Read the model definition and answer for the solid it produces. Units are mm, in the model's axes. Face numbers are marked on the shaded views. A direction names the side the tool comes from. Give positions to 0.01 mm unless a question says otherwise; leave off trailing zeros. Order: outer loops, then holes, each group sorted by start corner. A loop starts at its lowest first (then second) coordinate and runs counter-clockwise, first axis right, second up. Notation, with made-up numbers: (43.25, -39.5) - (69.25, -39.5) arc R27 ccw to (69.25, -22.5) - close; hole circle Ø8 at (-18, 22.25). An arc over 180 degrees is marked (long way). One line per item, written item: value. Start each with the question number.
```python
from build123d import *

# Parameters (mm, degrees)
SKETCH2_W               = 6.03
SKETCH2_H               = 7
BOSS_EXTRUDE1_DEPTH     = 15.64
CUT_EXTRUDE1_DEPTH      = 17.307968144
CUT_EXTRUDE1_DEPTH_BACK = 17.307968144
SKETCH3_W               = 4
SKETCH3_H               = 8.3
FILLET1_R               = 3.5
SKETCH4_R               = 1.5
BOSS_EXTRUDE2_DEPTH     = 4
CUT_EXTRUDE2_DEPTH      = 18.398270747
CUT_EXTRUDE2_DEPTH_BACK = 18.398270747
SKETCH7_W               = 7
SKETCH7_H               = 1.3
BOSS_EXTRUDE3_DEPTH     = 0.4
SKETCH8_R               = 1.75
BOSS_EXTRUDE4_DEPTH     = 21.14
SKETCH9_R               = 3.35
BOSS_EXTRUDE5_DEPTH     = 1.1
BOSS_EXTRUDE6_DEPTH     = 10.1
SKETCH11_R              = 3.35
BOSS_EXTRUDE7_DEPTH     = 1.1
SKETCH12_R              = 1.175
BOSS_EXTRUDE8_DEPTH     = 1
SKETCH13_R              = 1.25
BOSS_EXTRUDE9_DEPTH     = 1
CHAMFER1_SIZE           = 0.5
CHAMFER1_SIZE2          = 0.595876796
SKETCH14_R              = 2.55
BOSS_EXTRUDE10_DEPTH    = 0.5
CHAMFER3_SIZE           = 0.3


with BuildPart() as part:
    # Sketch2 → Boss-Extrude1 (new body)
    with BuildSketch(Plane(origin=(0, 0, 0), x_dir=(1, 0, 0), z_dir=(0, 1, 0))):
        Rectangle(SKETCH2_W, SKETCH2_H)
    extrude(amount=BOSS_EXTRUDE1_DEPTH)

    # Sketch3 → Cut-Extrude1 (cut, two sides: drawn at the far end of the back side and taken through both)
    with BuildSketch(Plane.XY.offset(-CUT_EXTRUDE1_DEPTH_BACK)):
        with Locations((0, 4.15)):
            Rectangle(SKETCH3_W, SKETCH3_H)
    extrude(amount=CUT_EXTRUDE1_DEPTH + CUT_EXTRUDE1_DEPTH_BACK, mode=Mode.SUBTRACT)

    # Fillet1
    fillet1_edges = [part.edges().sort_by_distance(p)[0] for p in [
        (-2.5075, 0, 3.5),
        (-2.5075, 0, -3.5),
        (2.5075, 0, -3.5),
        (2.5075, 0, 3.5),
    ]]
    fillet(fillet1_edges, radius=FILLET1_R - 0.0001)  # a hair under: the kernel refuses the full size

    # Sketch4 → Boss-Extrude2 (add)
    with BuildSketch(Plane(origin=(-2, 0, 0), x_dir=(0, 0, -1), z_dir=(1, 0, 0))):
        with Locations(Location((0, 2.4, 0), (0, 0, 180))):
            Circle(SKETCH4_R)
    extrude(amount=BOSS_EXTRUDE2_DEPTH)

    # Sketch6 → Cut-Extrude2 (cut, two sides: drawn at the far end of the back side and taken through both)
    with BuildSketch(Plane(origin=(0, 0, -3.5), x_dir=(-1, 0, 0), z_dir=(0, 0, -1)).offset(-CUT_EXTRUDE2_DEPTH_BACK)):
        with BuildLine():
            Line((-0.25, 13.4336972), (-0.25, 13.9336972))
            Line((-0.25, 13.9336972), (0.25, 13.9336972))
            Line((0.25, 13.9336972), (0.25, 13.4336972))
            ThreePointArc((0.25, 13.4336972), (0, 9.6), (-0.25, 13.4336972))
        make_face()
    extrude(amount=CUT_EXTRUDE2_DEPTH + CUT_EXTRUDE2_DEPTH_BACK, mode=Mode.SUBTRACT)

    # Sketch7 → Boss-Extrude3 (add)
    with BuildSketch(Plane(origin=(3.015, 0, 0), x_dir=(0, 0, -1), z_dir=(1, 0, 0))):
        with Locations((0, 14.6)):
            Rectangle(SKETCH7_W, SKETCH7_H)
        with Locations((0, 10.35)):
            Rectangle(SKETCH7_W, SKETCH7_H)
    boss_extrude3 = extrude(amount=BOSS_EXTRUDE3_DEPTH)

    # Mirror1: Boss-Extrude3 across plane
    add(boss_extrude3.mirror(Plane(origin=(0, 0, 0), x_dir=(0, 0, 1), z_dir=(1, 0, 0))))

    # Sketch8 → Boss-Extrude4 (add)
    with BuildSketch(Plane(origin=(0, 15.64, 0), x_dir=(1, 0, 0), z_dir=(0, 1, 0))):
        with Locations(Location((0, 0, 0), (0, 0, 270))):
            Circle(SKETCH8_R)
    extrude(amount=BOSS_EXTRUDE4_DEPTH)

    # Sketch9 → Boss-Extrude5 (add)
    with BuildSketch(Plane(origin=(0, 36.78, 0), x_dir=(1, 0, 0), z_dir=(0, 1, 0))):
        with Locations(Location((0, 0, 0), (0, 0, 270))):
            Circle(SKETCH9_R)
    extrude(amount=BOSS_EXTRUDE5_DEPTH)

    # Sketch10 → Boss-Extrude6 (add)
    with BuildSketch(Plane(origin=(0, 37.88, 0), x_dir=(1, 0, 0), z_dir=(0, 1, 0))):
        Polygon((-0.55, 2.3), (-0.55, 0.55), (-2.3, 0.55), (-2.3, -0.55), (-0.55, -0.55), (-0.55, -2.3), (0.55, -2.3), (0.55, -0.55), (2.3, -0.55), (2.3, 0.55), (0.55, 0.55), (0.55, 2.3), align=None)
    extrude(amount=BOSS_EXTRUDE6_DEPTH)

    # Sketch11 → Boss-Extrude7 (add)
    with BuildSketch(Plane(origin=(0, 47.98, 0), x_dir=(1, 0, 0), z_dir=(0, 1, 0))):
        with Locations(Location((0, 0, 0), (0, 0, 270))):
            Circle(SKETCH11_R)
    extrude(amount=BOSS_EXTRUDE7_DEPTH)

    # Sketch12 → Boss-Extrude8 (add)
    with BuildSketch(Plane(origin=(0, 49.08, 0), x_dir=(1, 0, 0), z_dir=(0, 1, 0))):
        with Locations(Location((0, 0, 0), (0, 0, 270))):
            Circle(SKETCH12_R)
    extrude(amount=BOSS_EXTRUDE8_DEPTH)

    # Sketch13 → Boss-Extrude9 (add)
    with BuildSketch(Plane(origin=(0, 50.08, 0), x_dir=(1, 0, 0), z_dir=(0, 1, 0))):
        with Locations(Location((0, 0, 0), (0, 0, 270))):
            Circle(SKETCH13_R)
    extrude(amount=BOSS_EXTRUDE9_DEPTH)

    # Chamfer1
    chamfer1_edges = [part.edges().sort_by_distance(p)[0] for p in [
        (0, 51.08, -1.25),
    ]]
    chamfer1_side = [part.faces().sort_by_distance(p)[0] for p in [
        (0, 50.58, -1.25),
    ]]
    chamfer(chamfer1_edges, length=CHAMFER1_SIZE, length2=CHAMFER1_SIZE2, reference=chamfer1_side[0])

    # Sketch14 → Boss-Extrude10 (add)
    with BuildSketch(Plane(origin=(0, 15.64, 0), x_dir=(1, 0, 0), z_dir=(0, 1, 0))):
        with Locations(Location((0, 0, 0), (0, 0, 90))):
            Circle(SKETCH14_R)
    extrude(amount=BOSS_EXTRUDE10_DEPTH)

    # Chamfer3
    chamfer3_edges = [part.edges().sort_by_distance(p)[0] for p in [
        (0, 16.14, -1.75),
        (0, 16.14, 2.55),
    ]]
    chamfer(chamfer3_edges, length=CHAMFER3_SIZE)


solid = part.part
```
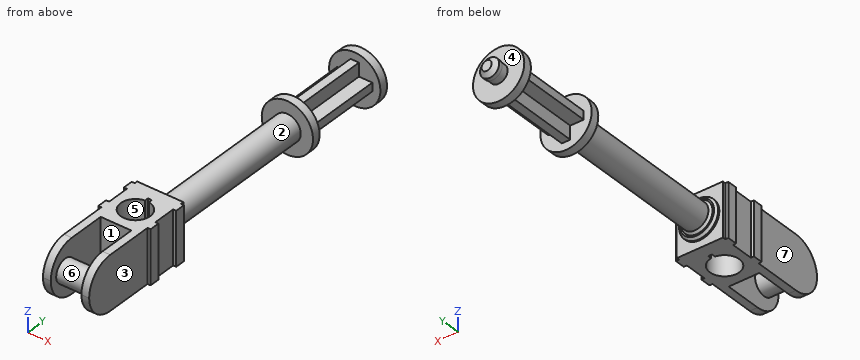
1) Section B-B on y = 40.5 is taken. Write down the section's boundary in (x, z).
2) Each of these flat-tipped pins is pushed along its axis until it touches: pin 1 (4 mm diameter, centred on x = -1.5, y = 44.5, fed in from +Z); pin 2 (2 mm diameter, centred on y = 5.5, z = 1, fed in from +X) (3 decimals); pin 3 (4 mm diameter, centred on y = 25.5, z = 0.5, fed in from +X). Where does it stop, or does it pass through?
3) The mould has two halves that part along X. Classify the marked faces 4, 5, 6 and 7: +X half, -X half, draft (parallel to the pull), parting line (faces both ways), or undercut.
4) Find the intervals of material crossed by probe 1 along X at (y, z) = (6.5, 2.75) (3 decimals); probe 2 along Y at (x, z) = (2.5, 1); probe 3 along Y at (x, z) = (-0.5, -2), in increasing order. Write a range as from..to.
5) Section A-A on y = 7 is taken. Write down the section's boundary in (x, z) (3 decimals), plus the area to 3 significant figures.
6) Section C-C on y = 21.5 is taken. Write down the section's boundary in (x, z).
7) For the marked faces 1, 2 and 3, determine the directions among +Z, -Z, +X, -X, +Y, -Y from which every point of the face is accessible in a straight line to the end or side of a thin tool.
Solved:
1. outline: (-2.3, -0.55) - (-0.55, -0.55) - (-0.55, -2.3) - (0.55, -2.3) - (0.55, -0.55) - (2.3, -0.55) - (2.3, 0.55) - (0.55, 0.55) - (0.55, 2.3) - (-0.55, 2.3) - (-0.55, 0.55) - (-2.3, 0.55) - close
2. pin 1: stops at z = 2.3
2. pin 2: stops at x = 3.015
2. pin 3: stops at x = 1.75
3. face 4: draft
3. face 5: undercut
3. face 6: undercut
3. face 7: -X half
4. probe 1: x = -3.015..-2, 2..3.015
4. probe 2: y = 0.15..15.64, 36.78..37.88, 47.98..49.08
4. probe 3: y = 8.3..9.67, 13.38..16.14, 36.78..49.08
5. outline: (-3.015, -3.5) - (-2, -3.5) - (-2, 3.5) - (-3.015, 3.5) - close; (2, -3.5) - (3.015, -3.5) - (3.015, 3.5) - (2, 3.5) - close
5. area: 14.2 mm2
6. outline: circle Ø3.5 at (0, 0)
7. face 1: +Z, -Z
7. face 2: none
7. face 3: +Z, -Z, +X, -Y
